Build history of the part. All positions in model axes, mm. A direction names the side the tool comes from. Round coordinates to 2 decimals unless told otherwise and drop trailing zeros. Loops run counter-clockwise (first coordinate to the right, second up) from the corner with the lowest first, then second, coordinate; pieces in that order, holes last.
from build123d import *

# Parameters (mm, degrees)
BOSS_EXTRUDE1_DEPTH = 10
SKETCH3_R           = 3.25
BOSS_EXTRUDE3_DEPTH = 10


with BuildPart() as part:
    # Sketch1 → Boss-Extrude1 (new body)
    with BuildSketch(Plane.XY):
        Polygon((57.505122166, 3.914590247), (24.739040394, -19.028467207), (24.739040394, -79.028467207), (32.850636148, -79.028467207), (32.850636148, -30.613026513), (65.616717919, -7.669969059), align=None)
    extrude(amount=BOSS_EXTRUDE1_DEPTH)

    # Sketch3 → Boss-Extrude3 (add)
    with BuildSketch(Plane(origin=(0, 0, 0), x_dir=(-1, 0, 0), z_dir=(0, 0, -1))):
        with Locations(Location((-55.41727971, -6.179512679, 0), (0, 0, 180))):
            Circle(SKETCH3_R)
        with Locations(Location((-28.794838271, -24.82074686, 0), (0, 0, 180))):
            Circle(SKETCH3_R)
    extrude(amount=BOSS_EXTRUDE3_DEPTH)


solid = part.part
(1) Slice it at A-A on x = 29. List the corners of the cut face in (y, z), plus the area to 3 significant figures.
Responses:
outline: (-79.03, 0) - (-28.06, 0) - (-28.06, -10) - (-21.58, -10) - (-21.58, 0) - (-16.04, 0) - (-16.04, 10) - (-79.03, 10) - close
area: 695 mm2
(2) Pin check, flat tips, straight feed: P1, Ø10, axis at y = -61, z = 2, coming from the +X side; P2, Ø6, axis at x = 43, z = 7, coming from the -Y side; P3, Ø6, axis at x = 58, z = 5, coming from the +Y side. Stop position of each tip, or through.
Responses:
P1: stops at x = 32.85
P2: stops at y = -25.61
P3: stops at y = 3.91
(3) Slice it at C-C on z = -1.25. List the corners of the cut face in (x, y), plus the area to 3 significant figures.
Responses:
outline: circle Ø6.5 at (28.79, -24.82); circle Ø6.5 at (55.42, -6.18)
area: 66.4 mm2
(4) Slice it at D-D on x = 56.5. List the corners of the cut face in (y, z).
Responses:
outline: (-14.05, 0) - (-9.24, 0) - (-9.24, -10) - (-3.12, -10) - (-3.12, 0) - (3.21, 0) - (3.21, 10) - (-14.05, 10) - close
(5) Slice it at B-B on y = -69. List the corners of the cut face in (x, z).
Responses:
outline: (24.74, 0) - (32.85, 0) - (32.85, 10) - (24.74, 10) - close
(6) Which spindle directions (+Z, -Z, +X, -X, +Y, -Y) get a long thin tool onto all of the face, cutting with end or side? Do faces 1 (the face through (32.851, -55, 5)), 2 (the face through (24.739, -49, 5)), 3 (the face through (25.548, -24.964, -4.93)). Say none if no direction does.
Responses:
face 1: +Z, -Z, +X, -Y
face 2: +Z, -Z, -X, +Y, -Y
face 3: -Z
(7) Probe line 1 (Z direction, x = 42, y = -18); line 2 (X direction, y = -42, z = 1); line 3 (Y direction, x = 49, z = 1.25). List the from-to ranges inside material, lowest first.
Responses:
line 1: z = 0 to 10
line 2: x = 24.74 to 32.85
line 3: y = -19.31 to -2.04
